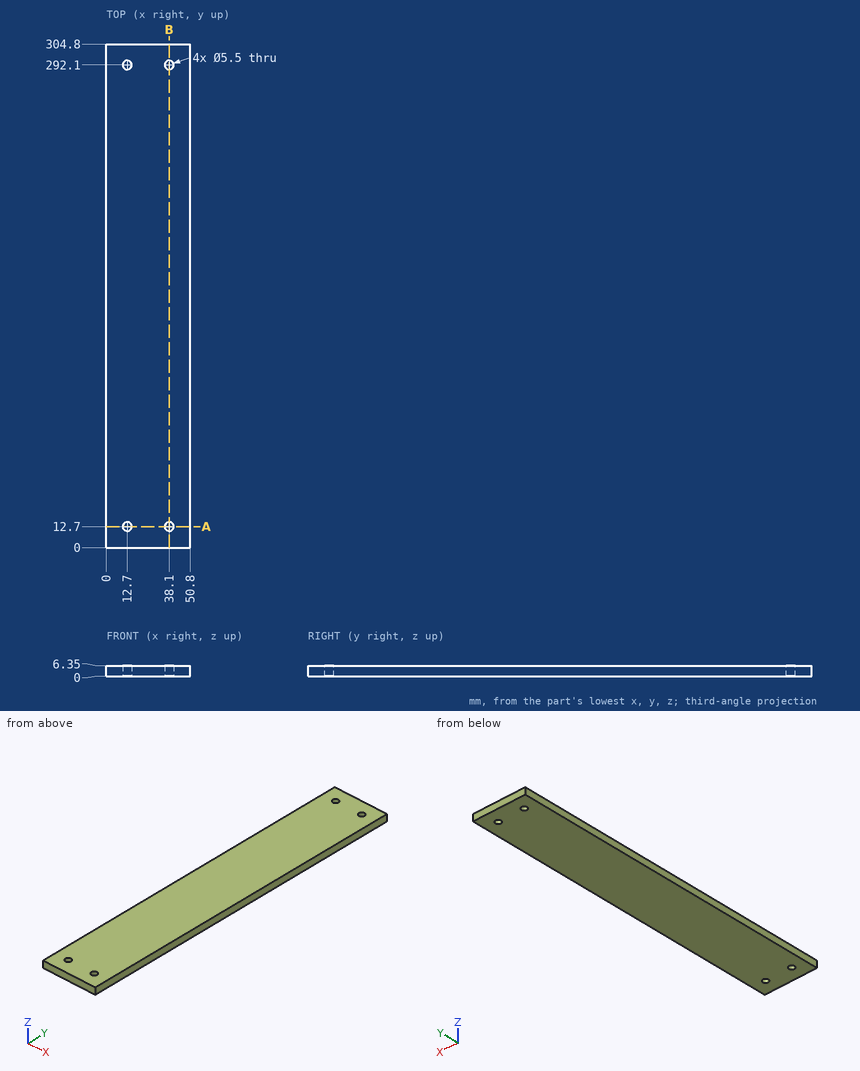
Here's the drawing with two shaded views (mm, measured from the low corner). I have some questions. Coordinates: 2 decimals unless noted, no trailing zeros. Order: outer loops, then holes, each group sorted by start corner. A loop starts at its lowest first (then second) coordinate and runs counter-clockwise, first axis right, second up.
Q1. Will these pins go through, and if not, where does the flat tip stop? pin 1 (9 mm diameter, centred on x = 12.7, y = 292.1, fed in from +Z); pin 2 (3.5 mm diameter, centred on x = 38.1, y = 12.7, fed in from -Z).
Q2. Please list where these lines run through material, in increasing order: L1, parallel to Y at x = 38.5, z = 2.75; L2, parallel to X at y = 292.1, z = 1.75; L3, parallel to Y at x = 40.5, z = 0.5.
Q3. Suppose I cut it at A-A on y = 12.7. Please give me the cut outline in (x, z).
Q4. Suppose I cut it at B-B on x = 38.1. Please give me the cut outline in (y, z), and give its area (3 significant figures).
Answer:
1. pin 1: stops at z = 6.35
1. pin 2: passes through
2. L1: y = 0 to 9.98, 15.42 to 289.38, 294.82 to 304.8
2. L2: x = 0 to 9.95, 15.45 to 35.35, 40.85 to 50.8
2. L3: y = 0 to 11.36, 14.04 to 290.76, 293.44 to 304.8
3. outline: (0, 0) - (9.95, 0) - (9.95, 6.35) - (0, 6.35) - close; (15.45, 0) - (35.35, 0) - (35.35, 6.35) - (15.45, 6.35) - close; (40.85, 0) - (50.8, 0) - (50.8, 6.35) - (40.85, 6.35) - close
4. outline: (0, 0) - (9.95, 0) - (9.95, 6.35) - (0, 6.35) - close; (15.45, 0) - (289.35, 0) - (289.35, 6.35) - (15.45, 6.35) - close; (294.85, 0) - (304.8, 0) - (304.8, 6.35) - (294.85, 6.35) - close
4. area: 1,870 mm2
